from build123d import *

# Parameters (mm, degrees)
F0_W     = 5
F0_H     = 68
F1_DEPTH = 10
F2_W     = 5
F2_H     = 5
F3_DEPTH = 30
F5_W     = 5
F5_H     = 5
F6_DEPTH = 5
F4_W     = 5
F4_H     = 5
F7_DEPTH = 5
F8_W     = 5
F8_H     = 6
F9_DEPTH = 5
F10_R    = 4.99999
F11_R    = 5


# Not quite as in the source:
# - a fillet or chamfer is up to 0.001 mm smaller than in the source, because OpenCascade refuses the exact size


with BuildPart() as f1:
    # F0 (on Top) → F1 (new body)
    with BuildSketch(Plane.XY):
        Rectangle(F0_W, F0_H)
    extrude(amount=F1_DEPTH)

    # F2 (on face) → F3 (join)
    with BuildSketch(Plane.XY.offset(10)):
        with Locations((0, 31.5)):
            Rectangle(F2_W, F2_H)
        with Locations((0, -31.5)):
            Rectangle(F2_W, F2_H)
    extrude(amount=F3_DEPTH)

    # F5 (on face) → F6 (join)
    with BuildSketch(Plane(origin=(0, -29, 0), x_dir=(-1, 0, 0), z_dir=(0, 1, 0))):
        with Locations((0, 37.5)):
            Rectangle(F5_W, F5_H)
    extrude(amount=F6_DEPTH)

    # F4 (on face) → F7 (join)
    with BuildSketch(Plane.XZ.offset(-29)):
        with Locations((0, 37.5)):
            Rectangle(F4_W, F4_H)
    extrude(amount=F7_DEPTH)

    # F8 (on face) → F9 (cut)
    with BuildSketch(Plane(origin=(0, 0, 0), x_dir=(1, 0, 0), z_dir=(0, 0, -1))):
        Rectangle(F8_W, F8_H)
    extrude(amount=-F9_DEPTH, mode=Mode.SUBTRACT)

    # F10 (radius 5 in the source; OpenCascade refuses exactly that, so slightly less here)
    f10_edges = [f1.edges().sort_by_distance(p)[0] for p in [
        (0, 24, 40),
        (0, -24, 40),
        (0, -34, 40),
    ]]
    fillet(f10_edges, radius=F10_R)

    # F11
    f11_edges = [f1.edges().sort_by_distance(p)[0] for p in [
        (0, 34, 40),
        (0, 34, 0),
        (0, -34, 0),
    ]]
    fillet(f11_edges, radius=F11_R)


solid = f1.part
The listing builds one solid part. Answer for the finished solid, in the listing's coordinates (mm). A direction names the side the tool comes from. Give positions to 0.01 mm unless a question says otherwise; leave off trailing zeros. Write each loop counter-clockwise with the first axis right and the second up, starting at its lowest first coordinate (ties: lowest second). Pieces come first, ordered by that corner, then holes.
Item 1: Determine the mould class of faces 6 (the cylindrical face through (0, -33, 2)), 7 (the flat face through (-2.5, 0, 6)), 8 (the flat face through (0, -3, 2)) for opening direction Y: released by +Y, released by -Y, zero draft, split by the parting line, or undercut.
Item 2: Section B-B, the plane z = 28.5 is taken. Write down the section's boundary in (x, y), plus the area to 3 significant figures.
Item 3: Find the intervals of material crossed by line 1 along Y through (x, z) = (-1.7, 18.5); line 2 along Z through (x, y) = (-1.55, 7); line 3 along Z through (x, y) = (-1.5, -25.5), in increasing order.
Item 4: Which of the six approach directions +Z, -Z, +X, -X, +Y, -Y give full straight-line access (tool end or side, diameter ignored) to faces 1 (the flat face through (0, -27, 35)), 2 (the cylindrical face through (0, -32, 39)), 3 (the flat face through (0, 0, 5)), 4 (the flat face through (0, -16, 0)), 5 (the cylindrical face through (0, 26, 39))?
Item 5: Section A-A, the plane y = 27 is taken. Write down the section's boundary in (x, z).
Item 6: Section D-D, the plane y = -13 is taken. Write down the section's boundary in (x, z), plus the area to 3 significant figures.
Item 7: Flat-ended cylindrical pins translate along their axes: P1, Ø1.5, axis at x = -0.5, y = 0.5, coming from the -Z side; P2, Ø1.5, axis at x = 0.5, z = 3, coming from the -Y side; P3, Ø2.5, axis at x = 1, y = 4, coming from the +Z side. Find the tip coordinate at first contact, or state that the pin passes through.
Completed:
1. face 6: released by -Y
1. face 7: zero draft
1. face 8: undercut
2. outline: (-2.5, -34) - (2.5, -34) - (2.5, -29) - (-2.5, -29) - close; (-2.5, 29) - (2.5, 29) - (2.5, 34) - (-2.5, 34) - close
2. area: 50.0 mm2
3. line 1: y = -34 to -29, 29 to 34
3. line 2: z = 0 to 10
3. line 3: z = 0 to 10, 35 to 38.57
4. face 1: +X, -X
4. face 2: +Z, +X, -X, -Y
4. face 3: -Z, +X, -X
4. face 4: -Z, +X, -X, +Y, -Y
4. face 5: +Z, +X, -X
5. outline: (-2.5, 0) - (2.5, 0) - (2.5, 10) - (-2.5, 10) - close; (-2.5, 35) - (2.5, 35) - (2.5, 39.58) - (-2.5, 39.58) - close
6. outline: (-2.5, 0) - (2.5, 0) - (2.5, 10) - (-2.5, 10) - close
6. area: 50.0 mm2
7. P1: stops at z = 5
7. P2: stops at y = -33.84
7. P3: stops at z = 10
